The model under review builds one solid part; all positions refer to its coordinate system, in mm. A direction names the side the tool comes from. Give positions to 0.01 mm unless a question says otherwise; leave off trailing zeros. Write each loop counter-clockwise with the first axis right and the second up, starting at its lowest first coordinate (ties: lowest second). Pieces come first, ordered by that corner, then holes.
from build123d import *

# Parameters (mm, degrees)
SKETCH1_R           = 32.625062454
BOSS_EXTRUDE1_DEPTH = 10
FILLET1_R           = 5
SKETCH2_W           = 9.918534818
SKETCH2_H           = 10.237019881
CUT_EXTRUDE1_DEPTH  = 10


with BuildPart() as part:
    # Sketch1 → Boss-Extrude1 (new body)
    with BuildSketch(Plane(origin=(0, 0, 0), x_dir=(1, 0, 0), z_dir=(0, 1, 0))):
        with Locations(Location((0, 0, 0), (0, 0, 270))):  # turned: the seam where the file's is
            Circle(SKETCH1_R)
    extrude(amount=BOSS_EXTRUDE1_DEPTH)

    # Fillet1
    fillet1_edges = [part.edges().sort_by_distance(p)[0] for p in [
        (0, 10, -32.625062454),
    ]]
    fillet(fillet1_edges, radius=FILLET1_R)

    # Sketch2 → Cut-Extrude1 (cut)
    with BuildSketch(Plane(origin=(0, 10, 0), x_dir=(1, 0, 0), z_dir=(0, 1, 0))):
        with Locations((4.959267409, 5.118509941)):
            Rectangle(SKETCH2_W, SKETCH2_H)
    extrude(amount=-CUT_EXTRUDE1_DEPTH, mode=Mode.SUBTRACT)


solid = part.part
1) To check wall thickness, follow probe 1 along Z at (x, y) = (1, 4); probe 2 along Z at (x, y) = (5.5, 0.5); probe 3 along Y at (x, z) = (28.5, -1). State the ranges of each line that lie inside material, in increasing order.
2) The part is to be moulded in two halves that separate along X. For faces 3 (the flat face through (5, 5, 0)), 4 (the flat face through (-6, 10, 0)), 5 (the cylindrical face through (-31.85, 2.46, -7.07)), say which applies: +X half, -X half, draft (parallel to the pull), parting line (faces both ways), or undercut.
3) Tool access review of faces 1 (the flat face through (0, 0, 7)), 2 (the flat face through (9.919, 5, -5)): name each direction out of +Z, -Z, +X, -X, +Y, -Y from which nothing blocks a thin tool from reaching the whole face with its end or side.
4) Insertion check: pin 1 (1.5 mm diameter, centred on y = 9, z = -17, fed in from -X); pin 2 (3 mm diameter, centred on y = 5, z = 19, fed in from +X); pin 3 (6 mm diameter, centred on y = 5, z = 19.5, fed in from -X); pin 4 (4 mm diameter, centred on x = -24.5, z = -14, fed in from +Y). Each pin has a flat end and moves straight along its axis. Give the tip position at first contact, or say it passes through.
5) Consider section A-A, the plane y = 7.75. Give the boundary of the cut face in (x, z).
Answer block:
1. probe 1: z = -32.61 to -10.24, 0 to 32.61
1. probe 2: z = -32.16 to -10.24, 0 to 32.16
1. probe 3: y = 0 to 9.92
2. face 3: undercut
2. face 4: draft
2. face 5: parting line
3. face 1: +Z, -Z, +X, -X, -Y
3. face 2: +Y, -Y
4. pin 1: stops at x = -26.56
4. pin 2: stops at x = 27.53
4. pin 3: stops at x = -28.15
4. pin 4: stops at y = 10
5. outline: circle Ø63.6 at (0, 0); hole (0, -10.24) - (9.92, -10.24) - (9.92, 0) - (0, 0) - close
